Geometry: see drawing. Coordinates: mm, zero at the bounding-box minimum. A direction names the side the tool comes from. Round coordinates to 2 decimals unless told otherwise and drop trailing zeros. Write each loop counter-clockwise with the first axis right and the second up, starting at its lowest first coordinate (ties: lowest second). Pieces come first, ordered by that corner, then holes. Notation, with made-up numbers: M 37,-24.5 L 80,-24.5 A20 ccw 80,9.5 Z; hole C 46.5,34.25 d9. An arc over 180 degrees is marked long. Write each question's results on one line, items separated by ' | '. Start each with the question number.
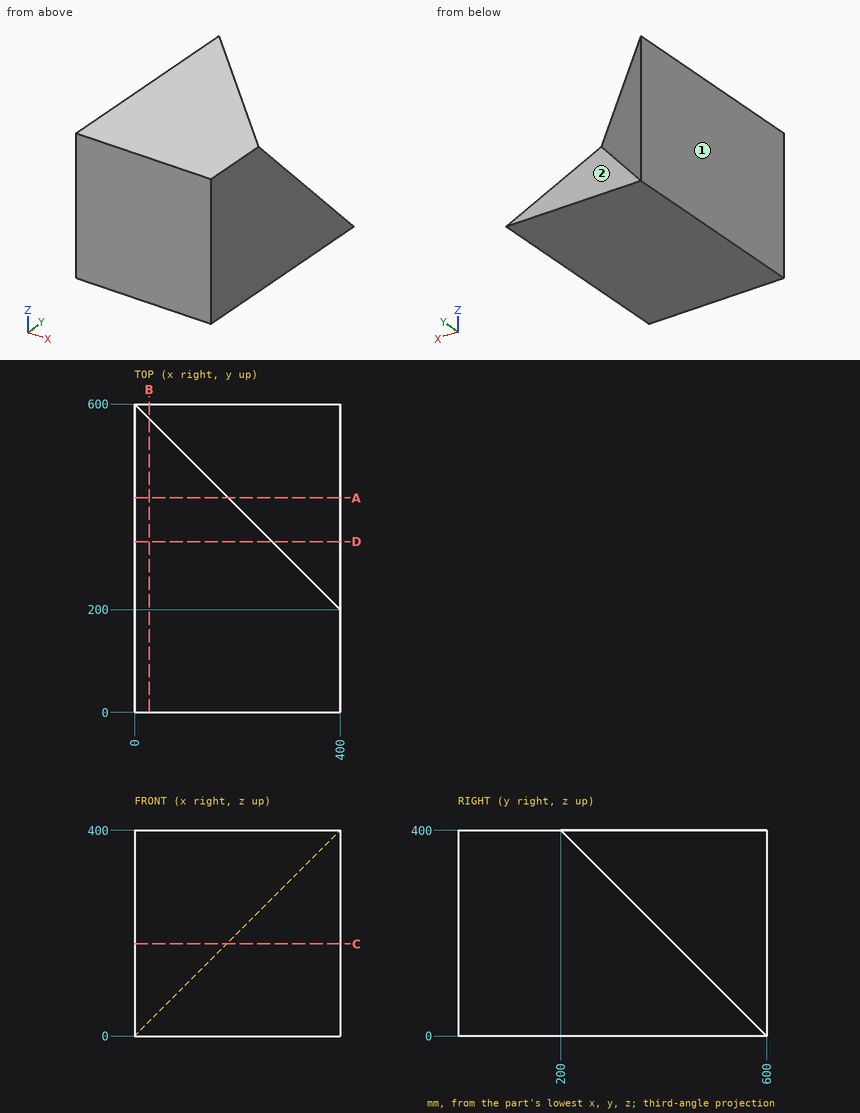
1. Line query: L1, parallel to Y at x = 364, z = 306.5; L2, parallel to Y at x = 377.5, z = 266.5; L3, parallel to X at y = 362, z = 353. Output: solid intervals per line, ascending. Write a range as from..to.
2. Cut plane B-B on x = 28.5. Output: boundary loops of the cut face in (y, z).
3. Access query for the marked faces 1 and 2. Directions: +Z, -Z, +X, -X, +Y, -Y. A direction counts if a zero-diameter tool reaches every point of the face in a straight line with its end or side. Return the directions, or none.
4. Cut plane A-A on y = 417.5. Output: boundary loops of the cut face in (x, z).
5. Cut plane C-C on z = 179. Output: boundary loops of the cut face in (x, y), and give its area (3 significant figures).
6. Cut plane D-D on y = 332. Output: boundary loops of the cut face in (x, z), and give its area (3 significant figures).
7. Contact query for flat-ended pins moving along their axis: P1, Ø12, axis at y = 418, z = 270.5, coming from the +X side; P2, Ø6, axis at x = 283, y = 523.5, coming from the +Z side; P3, Ø3, axis at x = 272, z = 217.5, coming from the +Y side. Output: stop coordinate, or through.
Answers follow:
1) L1: y = 0..293.5 | L2: y = 0..333.5 | L3: x = 0..238
2) outline: M 0,0 L 600,0 L 571.5,28.5 L 571.5,400 L 0,400 Z
3) face 1: +Z, -Z, -X, +Y, -Y | face 2: +Z, +X, +Y
4) outline: M 0,0 L 400,0 L 400,182.5 L 182.5,182.5 L 182.5,400 L 0,400 Z
5) outline: M 0,0 L 400,0 L 400,421 L 179,421 L 0,600 Z | area: 184,000 mm2
6) outline: M 0,0 L 400,0 L 400,268 L 268,268 L 268,400 L 0,400 Z | area: 143,000 mm2
7) P1: stops at x = 188 | P2: stops at z = 79.5 | P3: stops at y = 384
